The model under review builds one solid part; all positions refer to its coordinate system, in mm. Give positions to 0.01 mm unless a question says otherwise; leave off trailing zeros. Loops run counter-clockwise (first coordinate to the right, second up) from the corner with the lowest first, then second, coordinate; pieces in that order, holes last. Notation, with made-up numbers: M 80,88.5 L 99,88.5 A30 cw 99,117.5 Z; hole C -31.75,2 d9. An arc over 180 degrees is marked long. Return JSON: item names as keys, results as strings. Group by question number.
```python
from build123d import *

# Parameters (mm, degrees)
F0_R      = 5
F1_DEPTH  = 150
F1_FACE_R = 5
F0_R_2    = 7.5
F2_DEPTH  = 25
F3_R      = 7.7024133884
F3_R_2    = 5
F4_DEPTH  = 25


# Not quite as in the source:
# - a fillet or chamfer that OpenCascade refuses, or shapes differently, is made with other operations: its cross-section is extruded or revolved along the edge and cut away or added


with BuildPart() as f1:
    # F0 (on Front) → F1 (new body)
    with BuildSketch(Plane.XZ):
        Circle(F0_R)
    extrude(amount=-F1_DEPTH)

    # F1_face (on face) + F0 (on Front) → F2 (join)
    with BuildSketch(Plane.XZ):
        Circle(F1_FACE_R)
    with BuildSketch(Plane.XZ):
        Circle(F0_R_2)
        Circle(F0_R, mode=Mode.SUBTRACT)
    extrude(amount=F2_DEPTH)

    # F3 (on face) → F4 (join)
    with BuildSketch(Plane(origin=(0, 150, 0), x_dir=(-1, 0, 0), z_dir=(0, 1, 0))):
        Circle(F3_R)
        Circle(F3_R_2, mode=Mode.SUBTRACT)
        Circle(F3_R_2)
    extrude(amount=F4_DEPTH)

    # F5: fillet of radius 5 on 4 edges, made by hand

    # F5_s1 → F5_t2 (revolve, cut)
    with BuildSketch(Plane.XY):
        with BuildLine():
            ThreePointArc((7.5, -20), (6.0355339059, -23.5355339059), (2.5, -25))
            Line((2.5, -25), (7.5, -25))
            Line((7.5, -25), (7.5, -20))
        make_face()
    revolve(axis=Axis((0, -25, 0), (0, -1, 0)), mode=Mode.SUBTRACT)

    # F5_s3 → F5_t4 (revolve, cut)
    with BuildSketch(Plane.XY):
        with BuildLine():
            ThreePointArc((5, 0), (6.8301270189, -1.8301270189), (7.5, -4.3301270189))
            Line((7.5, -4.3301270189), (7.5, 0))
            Line((7.5, 0), (5, 0))
        make_face()
    revolve(axis=Axis((0, 0, 0), (0, -1, 0)), mode=Mode.SUBTRACT)

    # F5_s5 → F5_t6 (revolve, cut)
    with BuildSketch(Plane.XY):
        with BuildLine():
            ThreePointArc((-7.7024133884, 170), (-6.2379472943, 173.5355339059), (-2.7024133884, 175))
            Line((-2.7024133884, 175), (-7.7024133884, 175))
            Line((-7.7024133884, 175), (-7.7024133884, 170))
        make_face()
    revolve(axis=Axis((0, 175, 0), (0, 1, 0)), mode=Mode.SUBTRACT)

    # F5_s7 → F5_t8 (revolve, cut)
    with BuildSketch(Plane.XY):
        with BuildLine():
            ThreePointArc((-7.7024133884, 154.4408440371), (-6.9737090383, 151.8416069431), (-5, 150))
            Line((-5, 150), (-7.7024133884, 150))
            Line((-7.7024133884, 150), (-7.7024133884, 154.4408440371))
        make_face()
    revolve(axis=Axis((0, 150, 0), (0, 1, 0)), mode=Mode.SUBTRACT)


solid = f1.part
```
(1) Add section A-A (y = 46.5). Write out the cut boundary in (x, z), and give its area (3 significant figures).
(2) For probe 1 along Y at (x, z) = (6.5, 0); probe 2 along X at (y, z) = (65.5, 0.5); probe 3 along Y at (x, z) = (-4, -5) (3 decimals), list the stretches that pass through material, from the lowest coordinate up.
(3) Mouldability with a two-part tool opening along Y and no side actions: class faces 1 (the cylindrical face through (-7.115, 162.112, -2.95)), 2 (the flat face through (0, 175, 0)), 3 (the cylindrical face through (-1.08, 73.95, -4.88)), 4 (the flat face through (0, -25, 0)) as released by +Y, released by -Y, zero draft, split by the parting line, or undercut.
(4) For pin 1 (2 mm diameter, centred on y = 60.5, z = -5.5, fed in from +X); pin 2 (3 mm diameter, centred on x = 0.5, y = 115.5, fed in from -Z); pin 3 (1.5 mm diameter, centred on x = 4.5, y = 25, fed in from +Z), all flat-tipped, find the tip position at first contact; note any pin that passes through.
Verdict:
{
 "1": {"outline": "C 0,0 d10", "area": "78.5 mm²"},
 "2": {"probe 1": "y = -23 to -1.33, 151.19 to 173.25", "probe 2": "x = -4.97 to 4.97", "probe 3": "y = -23.125 to -1.205, 151.079 to 173.362"},
 "3": {"face 1": "zero draft", "face 2": "released by +Y", "face 3": "undercut", "face 4": "released by -Y"},
 "4": {"pin 1": "stops at x = 2.18", "pin 2": "stops at z = -5", "pin 3": "stops at z = 3.31"}
}
